Verification items for the finished model (mm, model axes). Face numbers are marked on the shaded views. A direction names the side the tool comes from. Give positions to 0.01 mm unless a question says otherwise; leave off trailing zeros. Write each loop counter-clockwise with the first axis right and the second up, starting at its lowest first coordinate (ties: lowest second). Pieces come first, ordered by that corner, then holes. Notation, with made-up numbers: (5.5, -37.5) -> (40.5, -37.5) arc R35 cw to (40.5, -1.5) -> close; hole circle Ø6 at (69.25, -4). An arc over 180 degrees is marked (long way). Answer as CSV lines item,"result". Start each with the question number.
1) Tool access check on the marked faces 1, 2 and 3. Record the directions out of +Z, -Z, +X, -X, +Y, -Y that give a thin tool (end or side, any length) a straight path to the whole face; none if there is none.
2) Gauge pin test, flat ends, axial feed: pin 1 Ø2 at (x, y) = (7.5, 0) entering from +Z; pin 2 Ø2 at (x, y) = (6, 3) entering from +Z. Record the tip position at first contact, or that the pin passes through.
3) Sectioned sample at C-C on y = 3. Record the cut outline in (x, z).
4) Mould release check, pull along Y, two halves, no side actions. Record for the marked faces 4, 5, 6 and 7: released by +Y, released by -Y, zero draft, split by the parting line, or undercut.
5) Material ranges on L1, parallel to X at y = 0, z = 3.5; L2, parallel to Z at x = 6, y = -2.5; L3, parallel to Y at x = 6.75, z = 2, recorded low to high.
6) Sectioned sample at B-B on z = 4.75. Record the cut outline in (x, y), and give its area (3 significant figures).
7) Sectioned sample at D-D on z = 2.5. Record the cut outline in (x, y).
8) Sectioned sample at A-A on x = 0. Record the cut outline in (y, z), and give its area (3 significant figures).
Autodesk Inventor part; units mm, degrees
ref_plane "YZ Plane" through (0, 0, 0) normal (1, 0, 0) x (0, 1, 0)
ref_plane "XZ Plane" through (0, 0, 0) normal (0, 1, 0) x (-1, 0, 0)
ref_plane "XY Plane" through (0, 0, 0) normal (0, 0, 1) x (1, 0, 0)
sketch "Skizze1" plane through (0, 0, 0) normal (0, 0, 1) x (1, 0, 0)
  line L0 (-14, 0) -> (14, 0)
  line L1 (0, -14) -> (0, 14)
  circle A0 centre (0, 0) radius 10
  circle A1 centre (0, 0) radius 2.5
  dimension "d0" = 5
  dimension "d1" = 20
extrude "Extrusion1" add sketch "Skizze1" along normal blind 5 contours A1 L1 A0 L0 | L0 A0 L1 A1 | A1 L0 A0 L1 | L1 A0 L0 A1
sketch "Skizze2" plane through (0, 0, 5) normal (0, 0, 1) x (1, 0, 0)
  circle A0 centre (0, 0) radius 10
  line L0 (-14, 0) -> (14, 0)
  line L1 (0, -14) -> (0, 14)
  line L2 (-7.1414, 7) -> (7.1414, 7)
  line L3 (7.1414, -7) -> (-7.1414, -7)
  dimension "d4" = 14
extrude "Extrusion2" cut sketch "Skizze2" against normal through all contours L2 L1 A0 | A0 L1 L3 | L1 L2 A0 | A0 L3 L1
sketch "Skizze3" plane through (-7.1414, 7, 5) normal (0, 1, 0) x (1, 0, 0)
  line L0 (0, 5) -> (14.2829, 5)
  line L1 (-6.8586, 5) -> (21.1414, 5)
  line L2 (7.1414, 6) -> (7.1414, -1)
  point P0 (7.1414, 5)
  point P1 (7.1414, 2.5)
  dimension "d7" = 2.5
hole "Bohrung1" at (0, 7, 2.5) direction (0, -1, 0) diameter 2.459 end up to surface
sketch "Skizze4" plane through (0, 0, 5) normal (0, 0, 1) x (1, 0, 0)
  circle A0 centre (0, 0) radius 2.5
  line L0 (-14, 0) -> (14, 0)
  line L1 (0, -14) -> (0, 14)
  circle A1 centre (0, 0) radius 7.5
  point P0 (-7.5, 0)
  point P1 (7.5, 0)
  dimension "d15" = 15
hole "Bohrung2" at (-7.5, 0, 5) at (7.5, 0, 5) direction (0, 0, -1) diameter 2.4 end through all countersink diameter 4.5 countersink angle 90
sketch "Skizze5" plane through (0, 0, 5) normal (0, 0, 1) x (1, 0, 0)
  circle A0 centre (0, 0) radius 2.5
  circle A1 centre (0, 0) radius 4
  dimension "d23" = 8
extrude "Extrusion3" add sketch "Skizze5" along normal blind 2
properties part number "13_1087_028"
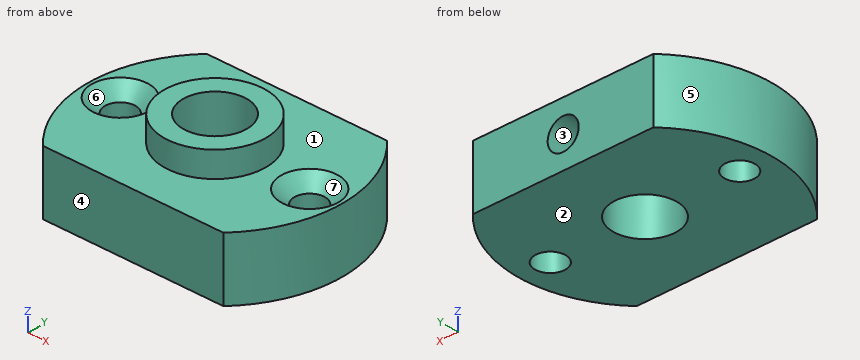
Ans:
1,face 1,"+Z"
1,face 2,"-Z, +X, -X, +Y, -Y"
1,face 3,"+Y"
2,pin 1,"passes through"
2,pin 2,"stops at z = 5"
3,outline,"(-9.54, 0) -> (9.54, 0) -> (9.54, 5) -> (2.65, 5) -> (2.65, 7) -> (-2.65, 7) -> (-2.65, 5) -> (-9.54, 5) -> close; hole circle Ø2.46 at (0, 2.5)"
4,face 4,"released by -Y"
4,face 5,"split by the parting line"
4,face 6,"undercut"
4,face 7,"undercut"
5,L1,"x = -10 to -8.7, -6.3 to -2.5, 2.5 to 6.3, 8.7 to 10"
5,L2,"z = 0 to 5"
5,L3,"y = -7 to -0.94, 0.94 to 7"
6,outline,"(-7.14, -7) -> (7.14, -7) arc R10 ccw to (7.14, 7) -> (-7.14, 7) arc R10 ccw to start; hole circle Ø4 at (-7.5, 0); hole circle Ø5 at (0, 0); hole circle Ø4 at (7.5, 0)"
6,area,"210 mm²"
7,outline,"(-7.14, -7) -> (7.14, -7) arc R10 ccw to (7.14, 7) -> (1.23, 7) -> (1.23, 2.18) arc R2.5 cw (long way) to (-1.23, 2.18) -> (-1.23, 7) -> (-7.14, 7) arc R10 ccw to start; hole circle Ø2.4 at (-7.5, 0); hole circle Ø2.4 at (7.5, 0)"
8,outline,"(-7, 0) -> (-2.5, 0) -> (-2.5, 7) -> (-4, 7) -> (-4, 5) -> (-7, 5) -> close; (2.5, 0) -> (7, 0) -> (7, 1.27) -> (2.5, 1.27) -> close; (2.5, 3.73) -> (7, 3.73) -> (7, 5) -> (4, 5) -> (4, 7) -> (2.5, 7) -> close"
8,area,"39.9 mm²"
